```python
from build123d import *

# Parameters (mm, degrees)
F0_R     = 2
F0_R_2   = 2.75
F1_DEPTH = 3
F2_R     = 11.75
F3_DEPTH = 2


with BuildPart() as f1:
    # F0 (on Top) → F1 (new body)
    with BuildSketch(Plane.XY):
        with BuildLine():
            Line((0, 25), (0, 0))
            Line((0, 0), (32, 0))
            Line((32, 0), (32, 25))
            ThreePointArc((32, 25), (16, 41), (0, 25))
        make_face()
        with Locations((16, 3.5)):
            Circle(F0_R, mode=Mode.SUBTRACT)
        with Locations((16, 35.5)):
            Circle(F0_R_2, mode=Mode.SUBTRACT)
    extrude(amount=F1_DEPTH)

    # F2 (on face) → F3 (cut)
    with BuildSketch(Plane.XY.offset(3)):
        with Locations((16, 19)):
            Circle(F2_R)
    extrude(amount=-F3_DEPTH, mode=Mode.SUBTRACT)


solid = f1.part
```
Can you work these out from the model? Positions are in its coordinate system, mm. A direction names the side the tool comes from. Coordinates: 2 decimals unless noted, no trailing zeros. Loops run counter-clockwise (first coordinate to the right, second up) from the corner with the lowest first, then second, coordinate; pieces in that order, holes last. Notation, with made-up numbers: (75, 11.5) -> (103, 11.5) arc R13 ccw to (103, 18.5) -> close; hole circle Ø3 at (-0.5, -39). An arc over 180 degrees is marked (long way). Answer as a JSON object with one key per item and string values.
1) Imagine slicing it at A-A (x = 16). Please give me the cut outline in (y, z), then the cut area to 3 significant figures.
Results:
{"outline": "(0, 0) -> (1.5, 0) -> (1.5, 3) -> (0, 3) -> close; (5.5, 0) -> (32.75, 0) -> (32.75, 3) -> (30.75, 3) -> (30.75, 1) -> (7.25, 1) -> (7.25, 3) -> (5.5, 3) -> close; (38.25, 0) -> (41, 0) -> (41, 3) -> (38.25, 3) -> close", "area": "47.5 mm^2"}
2) Thinking about a two-plate mould opening in Y: for faces 1 (the face through (16, 0, 1)), 2 (the face through (16, 19, 1)), 3 (the face through (32, 12, 1)), 4 (the face through (15.642, 38.227, 1.479)), which applies, pulls with the +Y half, pulls with the -Y half, needs draft (parallel to the pull), parting line crosses it, or undercut?
Results:
{"face 1": "pulls with the -Y half", "face 2": "undercut", "face 3": "needs draft", "face 4": "undercut"}
3) Imagine slicing it at C-C (z = 2.35). Please give me the cut outline in (x, y), then the cut area to 3 significant figures.
Results:
{"outline": "(0, 0) -> (32, 0) -> (32, 25) arc R16 ccw to (0, 25) -> close; hole circle Ø23.5 at (16, 19); hole circle Ø5.5 at (16, 35.5); hole circle Ø4 at (16, 3.5)", "area": "732 mm^2"}
4) For faces 5 (the face through (16, 21, 0)), 6 (the face through (4.26, 19.52, 2.01)), which set-ups out of +Z, -Z, +X, -X, +Y, -Y let a thin tool reach every point of the face, with its end or its side?
Results:
{"face 5": "-Z, +X, -X, +Y, -Y", "face 6": "+Z"}
5) For P1, Ø1, axis at x = 7.5, y = 24, coming from the +Z side; P2, Ø1, axis at x = 4, z = 2.5, coming from the +Y side, each with a flat end and sliding along its axis, tell me the tip position at first contact or that it passes through.
Results:
{"P1": "stops at z = 1", "P2": "stops at y = 36.12"}
6) Imagine slicing it at B-B (y = 3.5). Please give me the cut outline in (x, z), then the cut area to 3 significant figures.
Results:
{"outline": "(0, 0) -> (14, 0) -> (14, 3) -> (0, 3) -> close; (18, 0) -> (32, 0) -> (32, 3) -> (18, 3) -> close", "area": "84.0 mm^2"}
7) Imagine slicing it at D-D (y = 25.5). Please give me the cut outline in (x, z), then the cut area to 3 significant figures.
Results:
{"outline": "(0.01, 0) -> (31.99, 0) -> (31.99, 3) -> (25.79, 3) -> (25.79, 1) -> (6.21, 1) -> (6.21, 3) -> (0.01, 3) -> close", "area": "56.8 mm^2"}
8) If I drill on line 1 (Y direction, x = 16, z = 1.2); line 2 (Y direction, x = 16, z = 0.8); line 3 (Y direction, x = 14.5, z = 1.4), over which ranges is the centre line in solid material (lowest first)?
Results:
{"line 1": "y = 0 to 1.5, 5.5 to 7.25, 30.75 to 32.75, 38.25 to 41", "line 2": "y = 0 to 1.5, 5.5 to 32.75, 38.25 to 41", "line 3": "y = 0 to 2.18, 4.82 to 7.35, 30.65 to 33.2, 37.8 to 40.93"}
